The listing builds one solid part. Answer for the finished solid, in the listing's coordinates (mm). A direction names the side the tool comes from. Coordinates: 2 decimals unless noted, no trailing zeros. Write each loop counter-clockwise with the first axis right and the second up, starting at its lowest first coordinate (ties: lowest second). Pieces come first, ordered by that corner, then holes.
```python
from build123d import *

# Parameters (mm, degrees)
SKETCH1_W           = 17
SKETCH1_H           = 47
BOSS_EXTRUDE1_DEPTH = 6.581097747
CUT_EXTRUDE1_DEPTH  = 8
BOSS_EXTRUDE2_START = 8
BOSS_EXTRUDE2_DEPTH = 8
SKETCH4_W           = 39
SKETCH4_H           = 17
BOSS_EXTRUDE3_DEPTH = 35.070363466
SKETCH5_W           = 47
SKETCH5_H           = 17
BOSS_EXTRUDE4_DEPTH = 18.348538787
BOSS_EXTRUDE5_START = 8
BOSS_EXTRUDE5_DEPTH = 8
CUT_EXTRUDE2_DEPTH  = 3
CUT_EXTRUDE3_DEPTH  = 10
SKETCH9_W           = 9.5
SKETCH9_H           = 19
CUT_EXTRUDE4_DEPTH  = 45.598206242
SKETCH10_W          = 9.5
SKETCH10_H          = 19
CUT_EXTRUDE5_DEPTH  = 45.598206242
SKETCH11_W          = 5.9
SKETCH11_H          = 3.4
CUT_EXTRUDE6_DEPTH  = 45.598206242
SKETCH12_W          = 5.9
SKETCH12_H          = 3.4
CUT_EXTRUDE7_DEPTH  = 45.598206242
SKETCH13_W          = 5.9
SKETCH13_H          = 3.4
CUT_EXTRUDE8_DEPTH  = 45.598206242
CUT_EXTRUDE9_REACH  = 61.346
CUT_EXTRUDE10_DEPTH = 46.793012567
CUT_EXTRUDE11_DEPTH = 46.793012567
SKETCH17_W          = 5.9
SKETCH17_H          = 3.4
CUT_EXTRUDE12_DEPTH = 45.598206242
CUT_EXTRUDE13_REACH = 55.235
SKETCH19_W          = 6
SKETCH19_H          = 14
HOLE1_D             = 4.2
HOLE1_DEPTH         = 17.000025


with BuildPart() as part:
    # Sketch1 → Boss-Extrude1 (new body)
    with BuildSketch(Plane(origin=(-9.651461213, 0, 0), x_dir=(0, -1, 0), z_dir=(-1, 0, 0))):
        with Locations((8.5, -2.5)):
            Rectangle(SKETCH1_W, SKETCH1_H)
    extrude(amount=-BOSS_EXTRUDE1_DEPTH)

    # Sketch2 → Cut-Extrude1 (cut)
    with BuildSketch(Plane(origin=(0, 0, -26), x_dir=(-1, 0, 0), z_dir=(0, 0, -1))):
        with BuildLine():
            Line((3.070363466, 0), (3.070363466, -17))
            Line((3.070363466, -17), (9.651461213, -17))
            Line((9.651461213, -17), (9.651461213, -8.859566716))
            ThreePointArc((9.651461213, -8.859566716), (9.032439772, -5.88096289), (7.364540596, -3.336678977))
            Line((7.364540596, -3.336678977), (4.142347163, 0))
            Line((4.142347163, 0), (3.070363466, 0))
        make_face()
    extrude(amount=-CUT_EXTRUDE1_DEPTH, mode=Mode.SUBTRACT)

    # Sketch3 → Boss-Extrude2 (add)
    with BuildSketch(Plane(origin=(0, 0, -18), x_dir=(-1, 0, 0), z_dir=(0, 0, -1)).offset(BOSS_EXTRUDE2_START)):
        with BuildLine():
            Line((9.651461213, -9.140433284), (9.651461213, -17))
            Line((9.651461213, -17), (3.070363466, -17))
            ThreePointArc((3.070363466, -17), (7.750733238, -14.233963642), (9.651461213, -9.140433284))
        make_face()
    extrude(amount=-BOSS_EXTRUDE2_DEPTH)

    # Sketch4 → Boss-Extrude3 (add)
    with BuildSketch(Plane(origin=(-3.070363466, 0, 0), x_dir=(0, 0, -1), z_dir=(1, 0, 0))):
        with Locations((-1.5, -8.5)):
            Rectangle(SKETCH4_W, SKETCH4_H)
    extrude(amount=BOSS_EXTRUDE3_DEPTH)

    # Sketch5 → Boss-Extrude4 (add)
    with BuildSketch(Plane.ZY.offset(9.651461213)):
        with Locations((-2.5, -8.5)):
            Rectangle(SKETCH5_W, SKETCH5_H)
    extrude(amount=BOSS_EXTRUDE4_DEPTH)

    # Sketch6 → Boss-Extrude5 (add)
    with BuildSketch(Plane(origin=(0, 0, -18), x_dir=(-1, 0, 0), z_dir=(0, 0, -1)).offset(BOSS_EXTRUDE5_START)):
        with BuildLine():
            Line((-32, -17), (-32, 0))
            Line((-32, 0), (-1.142347163, 0))
            Line((-1.142347163, 0), (-4.364540596, -3.336678977))
            ThreePointArc((-4.364540596, -3.336678977), (-6.277598276, -11.444382635), (-0.070363466, -17))
            Line((-0.070363466, -17), (-32, -17))
        make_face()
    extrude(amount=-BOSS_EXTRUDE5_DEPTH)

    # Sketch7 → Cut-Extrude2 (cut)
    with BuildSketch(Plane(origin=(0, 0, 0), x_dir=(-1, 0, 0), z_dir=(0, 1, 0))):
        with BuildLine():
            Line((11.5, -11.5), (11.5, -7.745966692))
            ThreePointArc((11.5, -7.745966692), (17.5, 0), (11.5, 7.745966692))
            Line((11.5, 7.745966692), (11.5, 11.5))
            Line((11.5, 11.5), (-16.5, 11.5))
            Line((-16.5, 11.5), (-16.5, -11.5))
            Line((-16.5, -11.5), (11.5, -11.5))
        make_face()
    extrude(amount=-CUT_EXTRUDE2_DEPTH, mode=Mode.SUBTRACT)

    # Sketch8 → Cut-Extrude3 (cut)
    with BuildSketch(Plane(origin=(0, -3, 0), x_dir=(-1, 0, 0), z_dir=(0, 1, 0))):
        with BuildLine():
            Line((-3.5, -5.916079783), (8.166666667, -7.888106377))
            ThreePointArc((8.166666667, -7.888106377), (17.5, 0), (8.166666667, 7.888106377))
            Line((8.166666667, 7.888106377), (-3.5, 5.916079783))
            ThreePointArc((-3.5, 5.916079783), (3.5, 0), (-3.5, -5.916079783))
        make_face()
    extrude(amount=-CUT_EXTRUDE3_DEPTH, mode=Mode.SUBTRACT)

    # Sketch9 → Cut-Extrude4 (cut, through all)
    with BuildSketch(Plane.XZ.offset(17)):
        with Locations((27.25, 11.5)):
            Rectangle(SKETCH9_W, SKETCH9_H)
    extrude(amount=-CUT_EXTRUDE4_DEPTH, mode=Mode.SUBTRACT)

    # Sketch10 → Cut-Extrude5 (cut, through all)
    with BuildSketch(Plane.XZ.offset(17)):
        with Locations((-23.25, 11.5)):
            Rectangle(SKETCH10_W, SKETCH10_H)
    extrude(amount=-CUT_EXTRUDE5_DEPTH, mode=Mode.SUBTRACT)

    # Sketch11 → Cut-Extrude6 (cut, through all)
    with BuildSketch(Plane.XZ.offset(17)):
        with Locations((-13.25, 15.5)):
            Rectangle(SKETCH11_W, SKETCH11_H)
    extrude(amount=-CUT_EXTRUDE6_DEPTH, mode=Mode.SUBTRACT)

    # Sketch12 → Cut-Extrude7 (cut, through all)
    with BuildSketch(Plane.XZ.offset(17)):
        with Locations((16.75, 15.5)):
            Rectangle(SKETCH12_W, SKETCH12_H)
    extrude(amount=-CUT_EXTRUDE7_DEPTH, mode=Mode.SUBTRACT)

    # Sketch13 → Cut-Extrude8 (cut, through all)
    with BuildSketch(Plane.XZ.offset(17)):
        with Locations((16.75, -15.5)):
            Rectangle(SKETCH13_W, SKETCH13_H)
    extrude(amount=-CUT_EXTRUDE8_DEPTH, mode=Mode.SUBTRACT)

    # Cut-Extrude9: up to this plane
    cut_extrude9_end = Plane(origin=(-8.166666667, -13, 7.888106377), z_dir=(0.16666666666666724, 0, 0.9860132971832694))
    # Sketch14 → Cut-Extrude9 (cut, up to the surface)
    with BuildSketch(Plane.XY.offset(21), mode=Mode.PRIVATE) as cut_extrude9_sk1:
        with BuildLine():
            Line((-0.061320399, -7.610683259), (-1.5, -6.120886921))
            Line((-1.5, -6.120886921), (-2.938679601, -7.610683259))
            ThreePointArc((-2.938679601, -7.610683259), (-1.5, -11), (-0.061320399, -7.610683259))
        make_face()
    cut_extrude9_tool1 = split(extrude(cut_extrude9_sk1.sketch, amount=-CUT_EXTRUDE9_REACH, mode=Mode.PRIVATE), bisect_by=cut_extrude9_end, keep=Keep.BOTH, mode=Mode.PRIVATE)
    add(cut_extrude9_tool1.solids().sort_by_distance((-1.5, -8.847599, 21))[0], mode=Mode.SUBTRACT)

    # Sketch15 → Cut-Extrude10 (cut, through all)
    with BuildSketch(Plane.XY.offset(2)):
        with BuildLine():
            Line((-21.417452439, -6.971751585), (-23, -5.332975613))
            Line((-23, -5.332975613), (-24.582547561, -6.971751585))
            ThreePointArc((-24.582547561, -6.971751585), (-23, -10.7), (-21.417452439, -6.971751585))
        make_face()
    extrude(amount=-CUT_EXTRUDE10_DEPTH, mode=Mode.SUBTRACT)

    # Sketch16 → Cut-Extrude11 (cut, through all)
    with BuildSketch(Plane.XY.offset(2)):
        with BuildLine():
            Line((28.582547561, -6.971751585), (27, -5.332975613))
            Line((27, -5.332975613), (25.417452439, -6.971751585))
            ThreePointArc((25.417452439, -6.971751585), (27, -10.7), (28.582547561, -6.971751585))
        make_face()
    extrude(amount=-CUT_EXTRUDE11_DEPTH, mode=Mode.SUBTRACT)

    # Sketch17 → Cut-Extrude12 (cut, through all)
    with BuildSketch(Plane.XZ.offset(17)):
        with Locations((-13.25, -15.5)):
            Rectangle(SKETCH17_W, SKETCH17_H)
    extrude(amount=-CUT_EXTRUDE12_DEPTH, mode=Mode.SUBTRACT)

    # Cut-Extrude13: up to this plane
    cut_extrude13_end = Plane(origin=(3.5, -13, -5.916079783), z_dir=(0.1666666666666663, 0, -0.9860132971832695))
    # Sketch18 → Cut-Extrude13 (cut, up to the surface)
    with BuildSketch(Plane(origin=(0, 0, -18), x_dir=(-1, 0, 0), z_dir=(0, 0, -1)), mode=Mode.PRIVATE) as cut_extrude13_sk1:
        with BuildLine():
            Line((1.5, -6.120886921), (0.061320399, -7.610683259))
            ThreePointArc((0.061320399, -7.610683259), (1.5, -11), (2.938679601, -7.610683259))
            Line((2.938679601, -7.610683259), (1.5, -6.120886921))
        make_face()
    cut_extrude13_tool1 = split(extrude(cut_extrude13_sk1.sketch, amount=-CUT_EXTRUDE13_REACH, mode=Mode.PRIVATE), bisect_by=cut_extrude13_end, keep=Keep.BOTH, mode=Mode.PRIVATE)
    add(cut_extrude13_tool1.solids().sort_by_distance((-1.5, -8.847599, -18))[0], mode=Mode.SUBTRACT)

    # Sketch19 → Cut-Revolve1 (revolve, cut)
    with BuildSketch(Plane.XY, mode=Mode.PRIVATE) as cut_revolve1_sk:
        with Locations((5.5, -10)):
            Rectangle(SKETCH19_W, SKETCH19_H)
    revolve(cut_revolve1_sk.sketch.rotate(Axis((2.5, -3, 0), (0, -1, 0)), 270), axis=Axis((2.5, -3, 0), (0, -1, 0)), mode=Mode.SUBTRACT)

    # Hole1
    with Locations(Plane.XZ.offset(17)):
        with Locations((-9.5, 0)):
            Hole(HOLE1_D / 2, depth=HOLE1_DEPTH)


solid = part.part
```
(1) Section B-B, the plane z = 0 is taken. Write down the section's boundary in (x, y).
(2) Section A-A, the plane z = 14.5 is taken. Write down the section's boundary in (x, y), plus the area to 3 significant figures.
(3) Find the intervals of material crossed by probe 1 along X at (y, z) = (-3.25, 17); probe 2 along Z at (x, y) = (17, -7.75); probe 3 along X at (y, z) = (-2.25, -10), in increasing order.
(4) Each of these flat-tipped pins is pushed along its axis until it touches: pin 1 (6.5 mm diameter, centred on x = -9.5, z = 0, fed in from +Y); pin 2 (1.7 mm diameter, centred on y = -10, z = 15.5, fed in from -X); pin 3 (1 mm diameter, centred on x = -11, z = -19.5, fed in from +Y); pin 4 (1 mm diameter, centred on y = -8, z = 15.5, fed in from +X). Where does it stop, or does it pass through?
(5) Section D-D, the plane x = 2.5 is taken. Write down the section's boundary in (y, z), plus the area to 3 significant figures.
(6) Section C-C, the plane z = -16 is taken. Write down the section's boundary in (x, y), plus the area to 3 significant figures.
(7) Which of the six approach directions +Z, -Z, +X, -X, +Y, -Y give full straight-line access (tool end or side, diameter ignored) to faces 4 (the flat face through (-25.4, -8.6, 2)), 5 (the flat face through (16.5, -1, 0)), 6 (the flat face through (-10.3, -9, 15)), 7 (the flat face through (-22.2, -6.16, -11.8)), 8 (the flat face through (2.731, -1.645, -22.056))?
(8) For a pull along X with two mould halves and no side action, classify faces 1 (the flat face through (22.5, -9, 11)), 2 (the flat face through (17, -9, -13.8)), 3 (the flat face through (2, 0, -13)) as pulls with the +X half, pulls with the -X half, needs draft (parallel to the pull), parting line crosses it, or undercut.
Solution:
1. outline: (-28, -17) - (-11.6, -17) - (-11.6, -13) - (-17.5, -13) - (-17.5, 0) - (-28, 0) - close; (-7.4, -17) - (-3.5, -17) - (-3.5, -13) - (-7.4, -13) - close; (8.5, -17) - (32, -17) - (32, 0) - (16.5, 0) - (16.5, -3) - (8.5, -3) - close; hole (-24.58, -6.97) arc R2.2 ccw (long way) to (-21.42, -6.97) - (-23, -5.33) - close; hole (25.42, -6.97) arc R2.2 ccw (long way) to (28.58, -6.97) - (27, -5.33) - close
2. outline: (-18.5, -17) - (-16.2, -17) - (-16.2, 0) - (-18.5, 0) - close; (-10.3, -17) - (13.8, -17) - (13.8, 0) - (-10.3, 0) - close; (19.7, -17) - (22.5, -17) - (22.5, 0) - (19.7, 0) - close; hole (-2.94, -7.61) arc R2 ccw (long way) to (-0.06, -7.61) - (-1.5, -6.12) - close
2. area: 483 mm2
3. probe 1: x = -18.5 to -16.2, -10.3 to 13.8, 19.7 to 22.5
3. probe 2: z = -26 to -17.2, -13.8 to 13.8, 17.2 to 21
3. probe 3: x = -28 to -11.5, 16.5 to 32
4. pin 1: stops at y = -13
4. pin 2: stops at x = -18.5
4. pin 3: stops at y = 0
4. pin 4: stops at x = 22.5
5. outline: (-17, -26) - (-16.1, -26) - (-16.1, -18) - (-1.41, -18) - (-1.41, -26) - (0, -26) - (0, -11.5) - (-3, -11.5) - (-3, -6.09) - (-13, -6.09) - (-13, -6) - (-17, -6) - close; (-17, 6) - (-13, 6) - (-13, 6.09) - (-3, 6.09) - (-3, 11.5) - (0, 11.5) - (0, 21) - (-17, 21) - close
5. area: 443 mm2
6. outline: (-28, -17) - (-16.2, -17) - (-16.2, 0) - (-28, 0) - close; (-10.3, -17) - (13.8, -17) - (13.8, 0) - (-10.3, 0) - close; (19.7, -17) - (32, -17) - (32, 0) - (19.7, 0) - close; hole (-24.58, -6.97) arc R2.2 ccw (long way) to (-21.42, -6.97) - (-23, -5.33) - close; hole (-2.94, -7.61) arc R2 ccw (long way) to (-0.06, -7.61) - (-1.5, -6.12) - close; hole (25.42, -6.97) arc R2.2 ccw (long way) to (28.58, -6.97) - (27, -5.33) - close
6. area: 773 mm2
7. face 4: +Z, -X, +Y, -Y
7. face 5: +Y
7. face 6: +Y, -Y
7. face 7: +Z, -Z
7. face 8: -Z
8. face 1: pulls with the +X half
8. face 2: undercut
8. face 3: needs draft
